from build123d import *

# Parameters (mm, degrees)
SKETCH2_R           = 1.5
BOSS_EXTRUDE1_DEPTH = 3.5
CHAMFER1_SIZE       = 0.5


with BuildPart() as part:
    # Sketch1 → Revolve1 (revolve)
    with BuildSketch(Plane(origin=(0, 0, 0), x_dir=(1, 0, 0), z_dir=(0, 1, 0)), mode=Mode.PRIVATE) as revolve1_sk:
        with BuildLine():
            Line((0, 0), (-2, 0))
            Line((-2, 0), (-2, 6))
            Line((-2, 6), (-2.5, 6))
            ThreePointArc((-2.5, 6), (-1.530776406, 6.373105626), (-0.5, 6.5))
            Line((-0.5, 6.5), (0, 6.5))
            Line((0, 6.5), (0, 0))
        make_face()
    revolve(revolve1_sk.sketch.rotate(Axis((0, 0, 0), (0, 0, -1)), 180), axis=Axis((0, 0, 0), (0, 0, -1)))

    # Sketch2 → Boss-Extrude1 (add)
    with BuildSketch(Plane.XY):
        Circle(SKETCH2_R)
    extrude(amount=BOSS_EXTRUDE1_DEPTH)

    # Chamfer1
    chamfer1_edges = [part.edges().sort_by_distance(p)[0] for p in [
        (-1.5, 0, 3.5),
    ]]
    chamfer(chamfer1_edges, length=CHAMFER1_SIZE)


solid = part.part
The model under review builds one solid part; all positions refer to its coordinate system, in mm. A direction names the side the tool comes from. Give positions to 0.01 mm unless a question says otherwise; leave off trailing zeros. Write each loop counter-clockwise with the first axis right and the second up, starting at its lowest first coordinate (ties: lowest second). Pieces come first, ordered by that corner, then holes. Notation, with made-up numbers: M -12.5,25.5 L -3.5,25.5 A20 cw -3.5,52.5 Z; hole C 41.25,65 d6. An arc over 180 degrees is marked long. One line per question, with ' | ' between items. Start each with the question number.
Item 1: We need section A-A on z = -1.25. Write out the cut boundary in (x, y), plus the area to 3 significant figures.
Item 2: Wall thickness on line 1 (Z direction, x = -0.2, y = -0.55); line 2 (Z direction, x = -1.3, y = -0.05); line 3 (Y direction, x = -0.05, z = -3): over which ranges is each line inside the solid? List them lowest first. Write a range as from..to.
Item 3: For pin 1 (3 mm diameter, centred on y = 0, z = -1.5, fed in from -X); pin 2 (2 mm diameter, centred on y = 0.5, z = 1.5, fed in from +X); pin 3 (3 mm diameter, centred on y = -0.5, z = 2.5, fed in from -X), all flat-tipped, find the tip position at first contact; note any pin that passes through.
Item 4: For faces 1 (the flat face through (0, 0, -6.5)), 2 (the cylindrical face through (0, 2, -3)), list the 3-axis set-ups (+Z, -Z, +X, -X, +Y, -Y) from which the entire face can be reached by the end or side of a thin tool; tool diameter is ignored.
Results found:
1) outline: C 0,0 d4 | area: 12.6 mm2
2) line 1: z = -6.5..3.5 | line 2: z = -6.42..3.2 | line 3: y = -2..2
3) pin 1: stops at x = -2 | pin 2: stops at x = 1.5 | pin 3: stops at x = -1.5
4) face 1: -Z, +X, -X, +Y, -Y | face 2: +Z
